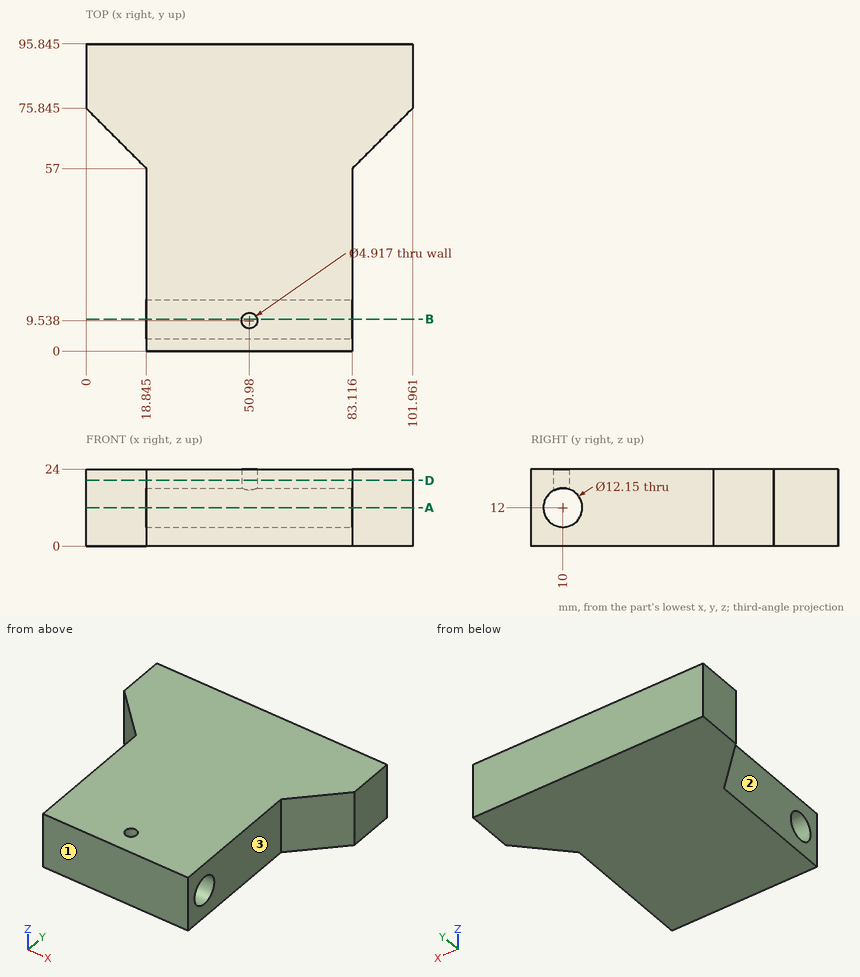
Study the drawing (mm; zero at the part's minimum x, y, z) and answer. A direction names the side the tool comes from. Coordinates: 2 decimals unless noted, no trailing zeros. Write each loop counter-clockwise with the first axis right and the second up, starting at its lowest first coordinate (ties: lowest second). Pieces come first, ordered by that corner, then holes. Notation, with made-up numbers: (53.5, 2) - (105.5, 2) arc R26 ccw to (105.5, 22) - close; hole circle Ø7 at (66.5, 52.5). An arc over 180 degrees is marked (long way). Answer as a JSON object with one key per item and string values.
Q1. Consider L1, parallel to Y at x = 39, z = 11.5 (1 decimal); L2, parallel to X at y = 41, z = 7.75 (1 decimal); L3, parallel to Z at x = 49, y = 10 (1 decimal). Determine where each line is inside the solid, lowest interval first. Write a range as from..to.
Results list:
{"L1": "y = 0..3.9, 16.1..95.8", "L2": "x = 18.8..83.1", "L3": "z = 0..5.9"}
Q2. Given pin 1 Ø3 at (x, z) = (16, 16) entering from -Y (1 decimal); pin 2 Ø3 at (y, z) = (52, 5) entering from +X; pin 3 Ø4.5 at (x, y) = (50.98, 9.54) entering from +Z, each flat-ended and moving along its own axis, determine where each tip first touches the part or whether it passes through.
Results list:
{"pin 1": "stops at y = 58.3", "pin 2": "stops at x = 83.12", "pin 3": "stops at z = 6.56"}
Q3. Find section D-D (z = 20.5). Write down the section's boundary in (x, y) (1 decimal), plus the area to 3 significant figures.
Results list:
{"outline": "(0, 75.8) - (18.8, 57) - (18.8, 0) - (83.1, 0) - (83.1, 57) - (102, 75.8) - (102, 95.8) - (0, 95.8) - close; hole circle Ø4.9 at (51, 9.5)", "area": "7,250 mm^2"}
Q4. Find section B-B (y = 10). Write down the section's boundary in (x, z) (1 decimal).
Results list:
{"outline": "(18.8, 0) - (83.1, 0) - (83.1, 5.9) - (18.8, 5.9) - close; (18.8, 18.1) - (48.6, 18.1) - (48.6, 24) - (18.8, 24) - close; (53.4, 18.1) - (83.1, 18.1) - (83.1, 24) - (53.4, 24) - close"}
Q5. Find section A-A (z = 12). Write down the section's boundary in (x, y) (1 decimal), plus the area to 3 significant figures.
Results list:
{"outline": "(0, 75.8) - (18.8, 57) - (18.8, 16.1) - (83.1, 16.1) - (83.1, 57) - (102, 75.8) - (102, 95.8) - (0, 95.8) - close; (18.8, 0) - (83.1, 0) - (83.1, 3.9) - (18.8, 3.9) - close", "area": "6,490 mm^2"}
Q6. Which of the six approach directions +Z, -Z, +X, -X, +Y, -Y give full straight-line access (tool end or side, diameter ignored) to the marked faces 1, 2 and 3?
Results list:
{"face 1": "+Z, -Z, +X, -X, -Y", "face 2": "+Z, -Z, -X, -Y", "face 3": "+Z, -Z, +X, -Y"}
